Source: CAD feature listing. Evaluate the final solid. Frame: model axes, mm. Round coordinates to 2 decimals unless told otherwise and drop trailing zeros. Order: outer loops, then holes, each group sorted by start corner. A loop starts at its lowest first (then second) coordinate and runs counter-clockwise, first axis right, second up. Notation, with made-up numbers: M -2,32.5 L 19,32.5 A6 cw 19,40.5 Z; hole C 6.5,68 d1. An arc over 180 degrees is marked long. Use one line per item in the form item = value. Start each with the question number.
Q1. Section B-B (x = 0). Return the cut outline in (y, z).
Q2. Section A-A (z = 1.2). Return the cut outline in (x, y).
Q3. Section C-C (y = -29.5). Return the cut outline in (x, z), plus the area to 3 significant figures.
Q4. Section D-D (y = -11.5). Return the cut outline in (x, z), plus the area to 3 significant figures.
Q5. Material intervals for probe 1 along Y at (x, z) = (0, 1.45); probe 2 along X at (y, z) = (-25.5, 2.5); probe 3 along X at (y, z) = (-28, 0.2), sorted ascending.
Q6. Contact query for flat-ended pins moving along their axis: pin 1 (4 mm diameter, centred on x = 0, y = -41.5, fed in from +Z); pin 2 (0.9 mm diameter, centred on y = -31, z = 1, fed in from +X). Output: stop coordinate, or through.
from build123d import *

# Parameters (mm, degrees)
SKETCH_1_R          = 21.25
EXTRUDE_1_DEPTH     = 3
SKETCH_2_R          = 1.6
CUT_EXTRUDE_1_DEPTH = 3
CUT_EXTRUDE_2_DEPTH = 54.359628934
FILLET_1_R          = 1.5
FILLET_2_R          = 3


with BuildPart() as part:
    # 草图1 → 凸台-拉伸1 (new body)
    with BuildSketch(Plane.XY):
        with BuildLine():
            Line((-26, 0), (-26, -46.5))
            Line((-26, -46.5), (26, -46.5))
            Line((26, -46.5), (26, 0))
            ThreePointArc((26, 0), (0, 26), (-26, 0))
        make_face()
        Circle(SKETCH_1_R, mode=Mode.SUBTRACT)
    extrude(amount=EXTRUDE_1_DEPTH)

    # 草图2 → 切除-拉伸1 (cut)
    with BuildSketch(Plane.XY.offset(3)):
        with Locations((0, -41.5)):
            Circle(SKETCH_2_R)
    extrude(amount=-CUT_EXTRUDE_1_DEPTH, mode=Mode.SUBTRACT)

    # 草图3 → 切除-拉伸2 (cut, through all)
    with BuildSketch(Plane.XY.offset(3)):
        Polygon((-26, -5.104538701), (-14.075326392, -46.5), (-26, -46.5), align=None)
        Polygon((26, -7.693867613), (10.888460039, -46.5), (26, -46.5), align=None)
        Polygon((-17.793337137, -18.847899848), (-2.05818452, -26.416707436), (-2.05818452, -35.688880127), (-9.759778205, -42.749397494), align=None)
        Polygon((17.129406646, -18.250362407), (2.589328912, -26.416707436), (2.589328912, -35.877249364), (9.228633813, -41.487929562), align=None)
    extrude(amount=-CUT_EXTRUDE_2_DEPTH, mode=Mode.SUBTRACT)

    # 圆角1
    fillet_1_edges = [part.edges().sort_by_distance(p)[0] for p in [
        (-9.759778205, -42.749397494, 1.5),
        (-17.793337137, -18.847899848, 1.5),
        (-2.05818452, -26.416707436, 1.5),
        (-2.05818452, -35.688880127, 1.5),
        (17.129406646, -18.250362407, 1.5),
        (9.228633813, -41.487929562, 1.5),
        (2.589328912, -35.877249364, 1.5),
        (2.589328912, -26.416707436, 1.5),
    ]]
    fillet(fillet_1_edges, radius=FILLET_1_R)

    # 圆角2
    fillet_2_edges = [part.edges().sort_by_distance(p)[0] for p in [
        (26, -7.693867613, 1.5),
        (10.888460039, -46.5, 1.5),
        (-26, -5.104538701, 1.5),
        (-14.075326392, -46.5, 1.5),
    ]]
    fillet(fillet_2_edges, radius=FILLET_2_R)


solid = part.part
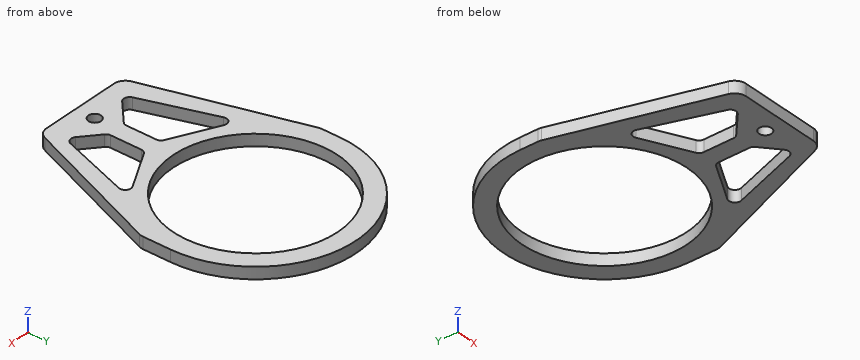
Results list:
q1.outline = M -46.5,0 L -43.1,0 L -43.1,3 L -46.5,3 Z; M -39.9,0 L -21.25,0 L -21.25,3 L -39.9,3 Z; M 21.25,0 L 26,0 L 26,3 L 21.25,3 Z
q2.outline = M -26,-4.68 A3 ccw -25.88,-5.51 L -14.7,-44.33 A3 ccw -11.82,-46.5 L 8.84,-46.5 A3 ccw 11.63,-44.59 L 25.8,-8.22 A3 ccw 26,-7.13 L 26,0 A26 ccw -26,0 Z; hole C 0,0 d42.5; hole M -16.66,-22.22 L -10.49,-40.56 A1.5 ccw -8.06,-41.19 L -2.54,-36.13 A1.5 ccw -2.06,-35.03 L -2.06,-27.36 A1.5 ccw -2.91,-26.01 L -14.59,-20.39 A1.5 ccw Z; hole C 0,-41.5 d3.2; hole M 2.59,-35.18 A1.5 ccw 3.12,-36.33 L 7.55,-40.07 A1.5 ccw 9.94,-39.41 L 15.87,-21.96 A1.5 ccw 13.71,-20.17 L 3.35,-25.99 A1.5 ccw 2.59,-27.29 Z
q3.outline = M -18.97,0 L -14.21,0 L -14.21,3 L -18.97,3 Z; M -2.06,0 L 2.59,0 L 2.59,3 L -2.06,3 Z; M 13.3,0 L 17.51,0 L 17.51,3 L 13.3,3 Z
q3.area = 40.8 mm2
q4.outline = M -24.16,0 L -17.87,0 L -17.87,3 L -24.16,3 Z; M 17.87,0 L 24.52,0 L 24.52,3 L 17.87,3 Z
q4.area = 38.8 mm2
q5.probe_1 = -46.5 to -43.1, -39.9 to -21.25, 21.25 to 26
q5.probe_2 = -20.12 to -15.56, -3.96 to 4.22, 14.66 to 19.07
q5.probe_3 = -19.4 to -14.72, -2.06 to 2.59, 13.81 to 18.09
q6.pin_1 = 3
q6.pin_2 = 17.1
